Build history of the part. All positions in model axes, mm. Face numbers are marked on the shaded views. A direction names the side the tool comes from. Round coordinates to 2 decimals unless told otherwise and drop trailing zeros. Loops run counter-clockwise (first coordinate to the right, second up) from the corner with the lowest first, then second, coordinate; pieces in that order, holes last.
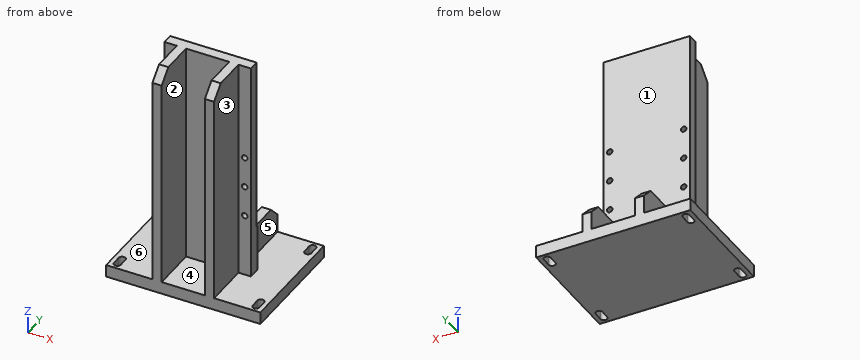
from build123d import *

# Parameters (mm, degrees)
F0_W     = 250
F0_H     = 190
F1_DEPTH = 20
F2_W     = 15
F2_H     = 73
F2_H_2   = 97
F3_DEPTH = 360
F4_W     = 3
F4_H     = 284.5591875911
F5_DEPTH = 140
F6_SIZE  = 20
F8_D     = 9


with BuildPart() as f1:
    # F0 (on Top) → F1 (new body)
    with BuildSketch(Plane.XY):
        Rectangle(F0_W, F0_H)
        with BuildLine():
            ThreePointArc((-107, -84.5), (-112.5, -90), (-118, -84.5))
            Line((-118, -84.5), (-118, -70.5))
            ThreePointArc((-118, -70.5), (-112.5, -65), (-107, -70.5))
            Line((-107, -70.5), (-107, -84.5))
        make_face(mode=Mode.SUBTRACT)
        with BuildLine():
            ThreePointArc((118, -84.5), (112.5, -90), (107, -84.5))
            Line((107, -84.5), (107, -70.5))
            ThreePointArc((107, -70.5), (112.5, -65), (118, -70.5))
            Line((118, -70.5), (118, -84.5))
        make_face(mode=Mode.SUBTRACT)
        with BuildLine():
            ThreePointArc((-118, 84.5), (-112.5, 90), (-107, 84.5))
            Line((-107, 84.5), (-107, 70.5))
            ThreePointArc((-107, 70.5), (-112.5, 65), (-118, 70.5))
            Line((-118, 70.5), (-118, 84.5))
        make_face(mode=Mode.SUBTRACT)
        with BuildLine():
            ThreePointArc((118, 70.5), (112.5, 65), (107, 70.5))
            Line((107, 70.5), (107, 84.5))
            ThreePointArc((107, 84.5), (112.5, 90), (118, 84.5))
            Line((118, 84.5), (118, 70.5))
        make_face(mode=Mode.SUBTRACT)
    extrude(amount=F1_DEPTH)

    # F2 (on face) → F3 (join)
    with BuildSketch(Plane.XY.offset(20)):
        with Locations((-42.5, -58.5)):
            Rectangle(F2_W, F2_H)
        with Locations((42.5, -58.5)):
            Rectangle(F2_W, F2_H)
        Polygon((-70, -22), (-50, -22), (-35, -22), (35, -22), (50, -22), (70, -22), (70, -2), (50, -2), (35, -2), (-35, -2), (-50, -2), (-70, -2), align=None)
        with Locations((42.5, 46.5)):
            Rectangle(F2_W, F2_H_2)
        with Locations((-42.5, 46.5)):
            Rectangle(F2_W, F2_H_2)
    extrude(amount=F3_DEPTH)

    # F4 (on face) → F5 (cut, symmetric)
    with BuildSketch(Plane.YZ.offset(50)):
        Polygon((-2, 70), (95, 70), (95, 380), (-2, 380), (-2, 95.4408124089), align=None)
        with Locations((-3.5, 237.7204062045)):
            Rectangle(F4_W, F4_H)
    extrude(amount=F5_DEPTH, both=True, mode=Mode.SUBTRACT)

    # F6
    f6_edges = [f1.edges().sort_by_distance(p)[0] for p in [
        (42.5, -95, 380),
        (-42.5, -95, 380),
        (42.5, 95, 70),
        (-42.5, 95, 70),
    ]]
    chamfer(f6_edges, length=F6_SIZE)

    # F8 (through all)
    with Locations(Plane.XZ.offset(22)):
        with Locations((-60, 222), (-60, 172), (-60, 122), (60, 222), (60, 172), (60, 122)):
            Hole(F8_D / 2)


solid = f1.part
(1) Slice it at A-A on z = 172. List the corners of the cut face in (x, y).
Responses:
outline: (-70, -22) - (-64.5, -22) - (-64.5, -5) - (-70, -5) - close; (-55.5, -22) - (-50, -22) - (-50, -95) - (-35, -95) - (-35, -22) - (35, -22) - (35, -95) - (50, -95) - (50, -22) - (55.5, -22) - (55.5, -5) - (-55.5, -5) - close; (64.5, -22) - (70, -22) - (70, -5) - (64.5, -5) - close
(2) Pull direction X, two halves, no side cores. Call the marked faces 4, 5 and 6: +X half, -X half, draft (parallel to the pull), parting line (faces both ways), or undercut.
Responses:
face 4: undercut
face 5: +X half
face 6: draft
(3) Slice it at C-C on y = 18. List the corners of the cut face in (x, z), plus the area to 3 significant figures.
Responses:
outline: (-125, 0) - (125, 0) - (125, 20) - (50, 20) - (50, 70) - (35, 70) - (35, 20) - (-35, 20) - (-35, 70) - (-50, 70) - (-50, 20) - (-125, 20) - close
area: 6,500 mm2
(4) Pin check, flat tips, straight feed: P1, Ø7, axis at x = 60, z = 172, coming from the +Y side; P2, Ø15, axis at y = 66.5, z = 48, coming from the +X side; P3, Ø6, axis at x = 42, z = 106, coming from the +Y side; P4, Ø2, axis at y = -55, z = 148.5, coming from the -X side. Stop position of each tip, or through.
Responses:
P1: passes through
P2: stops at x = 50
P3: stops at y = -5
P4: stops at x = -50
(5) Slice it at B-B on x = -112.5. List the corners of the cut face in (y, z).
Responses:
outline: (-95, 0) - (-90, 0) - (-90, 20) - (-95, 20) - close; (-65, 0) - (65, 0) - (65, 20) - (-65, 20) - close; (90, 0) - (95, 0) - (95, 20) - (90, 20) - close
(6) Which spindle directions (+Z, -Z, +X, -X, +Y, -Y) get a long thin tool onto all of the face, cutting with end or side? Do the marked faces 1, 2 and 3. Say none if no direction does.
Responses:
face 1: +Z, +X, -X, +Y
face 2: +Z, -Y
face 3: +Z, +X, -Y
(7) Slice it at D-D on z = 85. List the corners of the cut face in (x, y).
Responses:
outline: (-70, -22) - (-50, -22) - (-50, -95) - (-35, -95) - (-35, -22) - (35, -22) - (35, -95) - (50, -95) - (50, -22) - (70, -22) - (70, -2) - (-70, -2) - close
(8) Probe line 1 (Z direction, x = 60, y = -17); line 2 (X direction, y = -38.5, z = 140.5); line 3 (Z direction, x = 74.5, y = 19.5). List the from-to ranges inside material, lowest first.
Responses:
line 1: z = 0 to 117.5, 126.5 to 167.5, 176.5 to 217.5, 226.5 to 380
line 2: x = -50 to -35, 35 to 50
line 3: z = 0 to 20
